The listing builds one solid part. Answer for the finished solid, in the listing's coordinates (mm). A direction names the side the tool comes from. Coordinates: 2 decimals unless noted, no trailing zeros. Loops run counter-clockwise (first coordinate to the right, second up) from the corner with the lowest first, then second, coordinate; pieces in that order, holes last. Notation, with made-up numbers: (-34.75, 43) -> (8.25, 43) arc R12 ccw to (8.25, 59) -> close; hole circle Ø7 at (9.25, -6). An arc over 180 degrees is marked (long way). Answer in a Markdown table with one row per item.
```python
from build123d import *

# Parameters (mm, degrees)
ESQUISSE1_W                  = 20
ESQUISSE1_H                  = 40
BOSS_EXTRU_1_DEPTH           = 300
ENL_V_MAT_EXTRU_1_DEPTH      = 1
ENL_V_MAT_EXTRU_1_DEPTH_BACK = 41


with BuildPart() as part:
    # Esquisse1 → Boss.-Extru.1 (new body)
    with BuildSketch(Plane.XY):
        with Locations((10, 20)):
            Rectangle(ESQUISSE1_W, ESQUISSE1_H)
    extrude(amount=BOSS_EXTRU_1_DEPTH)

    # Esquisse2 → Enlèv. mat.-Extru.1 (cut, two sides)
    with BuildSketch(Plane.XZ) as enl_v_mat_extru_1_sk:
        Polygon((-551.479454827, 30), (0, 30), (10, 30), (10, 40), (0, 40), (-551.479454827, 40), (-1654.438364482, 40), (-1654.438364482, 30), align=None)
    extrude(amount=ENL_V_MAT_EXTRU_1_DEPTH, mode=Mode.SUBTRACT)
    extrude(enl_v_mat_extru_1_sk.sketch, amount=-ENL_V_MAT_EXTRU_1_DEPTH_BACK, mode=Mode.SUBTRACT)


solid = part.part
```
Item 1: A cutting plane is placed at B-B, the plane y = 3. Determine the outline of the cut face in (x, z), plus the area to 3 significant figures.
Findings below:
| item | result |
|---|---|
| outline | (0, 0) -> (20, 0) -> (20, 300) -> (0, 300) -> (0, 40) -> (10, 40) -> (10, 30) -> (0, 30) -> close |
| area | 5,900 mm2 |
Item 2: A tool of negligible diameter and unlimited length cuts with its end or side. For faces 1 (the face through (10, 40, 148)), 2 (the face through (10, 20, 35)), from which of +Z, -Z, +X, -X, +Y, -Y can it reach the whole face along a straight path? Write none if from no direction.
Findings below:
| item | result |
|---|---|
| face 1 | +Z, -Z, +X, -X, +Y |
| face 2 | -X, +Y, -Y |
Item 3: A flat-ended cylindrical pin translates along its axis: pin 1 Ø3 at (y, z) = (24, 34) entering from -X. Find the tip coordinate at first contact, or state that the pin passes through.
Findings below:
| item | result |
|---|---|
| pin 1 | stops at x = 10 |
Item 4: Determine the mould class of faces 3 (the face through (10, 20, 0)), 4 (the face through (0, 20, 15)), 5 (the face through (5, 20, 40)) for opening direction Z: +Z half, -Z half, draft (parallel to the pull), parting line (faces both ways), or undercut.
Findings below:
| item | result |
|---|---|
| face 3 | -Z half |
| face 4 | draft |
| face 5 | undercut |
Item 5: A cutting plane is placed at A-A, the plane x = 5.5. Determine the outline of the cut face in (y, z), plus the area to 3 significant figures.
Findings below:
| item | result |
|---|---|
| outline | (0, 0) -> (40, 0) -> (40, 30) -> (0, 30) -> close; (0, 40) -> (40, 40) -> (40, 300) -> (0, 300) -> close |
| area | 11,600 mm2 |
Item 6: Find the intervals of material crossed by probe 1 along Z at (x, y) = (8, 30), in increasing order.
Findings below:
| item | result |
|---|---|
| probe 1 | z = 0 to 30, 40 to 300 |
